Autodesk Inventor part; units mm, degrees
ref_plane "YZ Plane" through (0, 0, 0) normal (1, 0, 0) x (0, 1, 0)
ref_plane "XZ Plane" through (0, 0, 0) normal (0, 1, 0) x (-1, 0, 0)
ref_plane "XY Plane" through (0, 0, 0) normal (0, 0, 1) x (1, 0, 0)
sketch "Sketch1" plane through (0, 0, 0) normal (0, 1, 0) x (-1, 0, 0)
  line L0 (15, 20.25) -> (-15, 20.25)
  line L1 (-15, 20.25) -> (-15, -20.25)
  line L2 (-15, -20.25) -> (15, -20.25)
  line L3 (15, -20.25) -> (15, 20.25)
  point P0 (0, 0)
  point P1 (15, 0)
  point P2 (0, 20.25)
  dimension "d0" = 30
  dimension "d1" = 40.5
extrude "Plate1" add sketch "Sketch1" along normal blind 1.5
sketch "Sketch2" plane through (15, 0, 21.75) normal (0, 0, -1) x (-1, 0, 0)
  line L0 (30, 0) -> (0, 0)
  line L1 (0, 0) -> (0, 30)
  line L2 (0, 30) -> (30, 30)
  line L3 (30, 30) -> (30, 0)
edge flange "Flange1" height 30 angle 90 thickness 1.5 bend radius 0.31 thickness toward (0, 0, -1) relief tear relief width 1.5 relief depth 0.75 corner gap 0.31 corner form 0 edges at (0, 1.5, 20.25) (0, 1.5, -20.25) wall of the first edge with corners at (-15, 0, 21.75) (15, 0, 21.75) (15, 30, 21.75) (-15, 30, 21.75)
bend "Bend1"
corner "Corner1"
sketch "Sketch3" plane through (15, 30, -21.75) normal (0, 0, -1) x (-1, 0, 0)
  circle A0 centre (15, -20.82) radius 0.7835
  circle A1 centre (8, -13.52) radius 0.7835
  circle A2 centre (22, -13.52) radius 0.7835
  circle A3 centre (7, -0.3) radius 0.7835
  circle A4 centre (23, -0.3) radius 0.7835
  line L0 (21.07, -22.22) -> (8.93, -22.22)
  line L1 (21.07, -22.22) -> (21.07, -21.5)
  arc A5 (23.07, -19.5) -> (21.07, -21.5) centre (23.07, -21.5) ccw
  line L2 (23.07, -19.5) -> (23.79, -19.5)
  line L3 (23.79, 12.6) -> (23.79, -19.5)
  line L4 (23.79, 12.6) -> (23.07, 12.6)
  arc A6 (21.07, 14.6) -> (23.07, 12.6) centre (23.07, 14.6) ccw
  line L5 (21.07, 14.6) -> (21.07, 15.32)
  line L6 (8.93, 15.32) -> (21.07, 15.32)
  line L7 (8.93, 15.32) -> (8.93, 14.6)
  arc A7 (6.93, 12.6) -> (8.93, 14.6) centre (6.93, 14.6) ccw
  line L8 (6.93, 12.6) -> (6.21, 12.6)
  line L9 (6.21, -19.5) -> (6.21, 12.6)
  line L10 (6.21, -19.5) -> (6.93, -19.5)
  arc A8 (8.93, -21.5) -> (6.93, -19.5) centre (6.93, -21.5) ccw
  line L11 (8.93, -21.5) -> (8.93, -22.22)
  circle A9 centre (15, 6.6) radius 6.4
  point P0 (15, -30)
hole "Hole1" at (-7, 16.48, -21.75) at (0, 9.18, -21.75) at (7, 16.48, -21.75) direction (0, 0, 1) diameter 2.1 depth 1.5
equation "\"d18\" = Thickness"
equation "\"d2\" = Thickness"
equation "\"d3\" = BendReliefWidth"
equation "\"d4\" = BendReliefDepth"
equation "\"d5\" = MinimumRemnant"
equation "\"d6\" = TransitionRadius"
equation "\"d9\" = BendRadius"
equation "\"d10\" = CornerReliefSize"
equation "\"d11\" = GapSize"
equation "\"d12\" = JacobiRadiusSize"
equation "\"BendReliefWidth\" = Thickness"
equation "\"BendReliefDepth\" = 0.5 * Thickness"
equation "\"CornerReliefSize\" = 4 * Thickness"
equation "\"MinimumRemnant\" = 2 * Thickness"
equation "\"TransitionRadius\" = BendRadius"
equation "\"JacobiRadiusSize\" = BendRadius"
equation "\"GapSize\" = Thickness"
properties part number "chris" material "Aluminum 6061-AHC"
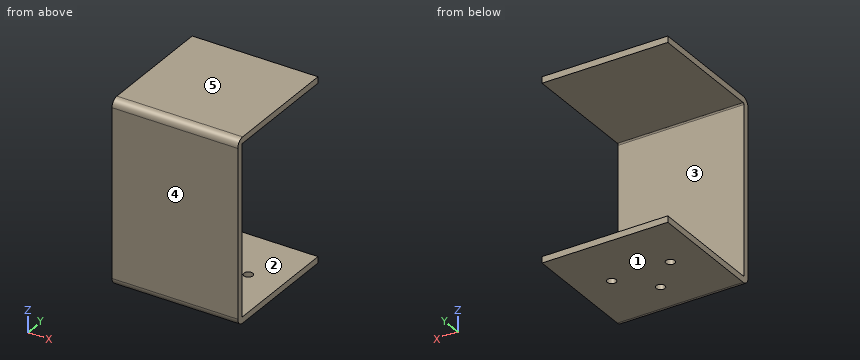
Source: CAD feature listing. Evaluate the final solid. Frame: model axes, mm. Face numbers are marked on the shaded views. A direction names the side the tool comes from. Round coordinates to 2 decimals unless told otherwise and drop trailing zeros. Loops run counter-clockwise (first coordinate to the right, second up) from the corner with the lowest first, then second, coordinate; pieces in that order, holes last. Notation, with made-up numbers: M 74.5,71 L 107.5,71 A14 ccw 107.5,92 Z; hole C -12.5,19 d8. An arc over 180 degrees is marked long. Return JSON: item names as keys, results as strings. Group by question number.
1. Section query D-D on y = 5. Output: boundary loops of the cut face in (x, z).
2. Section query B-B on x = 7. Output: boundary loops of the cut face in (y, z), and give its area (3 significant figures).
3. Section query C-C on y = 16.48. Output: boundary loops of the cut face in (x, z).
4. Section query A-A on y = 9.18. Output: boundary loops of the cut face in (x, z), and give its area (4 significant figures).
5. Reachability of the marked faces 1 and 2 from +Z, -Z, +X, -X, +Y, -Y: full face, straight path, thin tool, end or side. Return the list, or none.
6. Pin query (flat end, axial travel): pin 1 (6 mm diameter, centred on x = 4, z = -14.5, fed in from +Y); pin 2 (10 mm diameter, centred on x = 4.5, z = 13.5, fed in from -Y). Return the tip coordinate at first contact, or that it passes through.
7. Material intervals for line 1 along X through (y, z) = (16.48, -21.2); line 2 along Z through (x, y) = (4.75, 17.5); line 3 along X through (y, z) = (9.18, -20.7), sorted ascending. Write a range as from..to.
8. Mould query, pull axis Z, two halves, no side actions, for the marked faces 3, 4 and 5. Classes: released by +Z, released by -Z, zero draft, split by the parting line, or undercut.
Checks:
{
 "1": {"outline": "M -15,-21.75 L 15,-21.75 L 15,-20.25 L -15,-20.25 Z; M -15,20.25 L 15,20.25 L 15,21.75 L -15,21.75 Z"},
 "2": {"outline": "M 0,-19.94 A1.81 ccw 1.81,-21.75 L 15.43,-21.75 L 15.43,-20.25 L 1.81,-20.25 A0.31 cw 1.5,-19.94 L 1.5,19.94 A0.31 cw 1.81,20.25 L 30,20.25 L 30,21.75 L 1.81,21.75 A1.81 ccw 0,19.94 Z; M 17.53,-21.75 L 30,-21.75 L 30,-20.25 L 17.53,-20.25 Z", "area": "146 mm²"},
 "3": {"outline": "M -15,-21.75 L -8.05,-21.75 L -8.05,-20.25 L -15,-20.25 Z; M -15,20.25 L 15,20.25 L 15,21.75 L -15,21.75 Z; M -5.95,-21.75 L 5.95,-21.75 L 5.95,-20.25 L -5.95,-20.25 Z; M 8.05,-21.75 L 15,-21.75 L 15,-20.25 L 8.05,-20.25 Z"},
 "4": {"outline": "M -15,-21.75 L -1.05,-21.75 L -1.05,-20.25 L -15,-20.25 Z; M -15,20.25 L 15,20.25 L 15,21.75 L -15,21.75 Z; M 1.05,-21.75 L 15,-21.75 L 15,-20.25 L 1.05,-20.25 Z", "area": "86.85 mm²"},
 "5": {"face 1": "-Z, +X, -X, +Y, -Y", "face 2": "+X, -X, +Y"},
 "6": {"pin 1": "stops at y = 1.5", "pin 2": "stops at y = 0"},
 "7": {"line 1": "x = -15..-8.05, -5.95..5.95, 8.05..15", "line 2": "z = -21.75..-20.25, 20.25..21.75", "line 3": "x = -15..-1.05, 1.05..15"},
 "8": {"face 3": "undercut", "face 4": "zero draft", "face 5": "released by +Z"}
}
